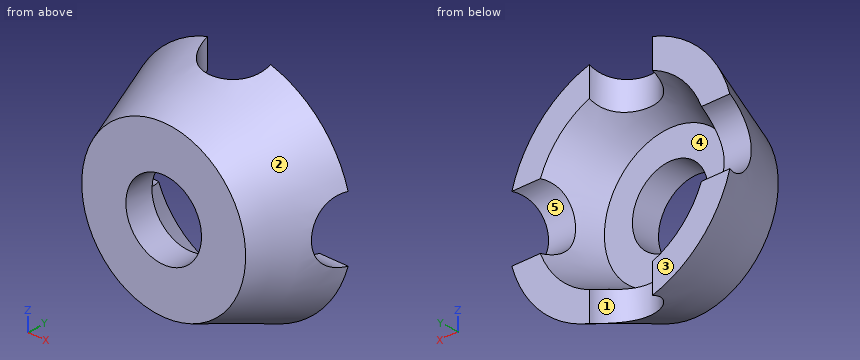
```python
from build123d import *

# Parameters (mm, degrees)
CUT_EXTRUDE1_DEPTH      = 58.166423712
CUT_EXTRUDE1_DEPTH_BACK = 58.166423712
SKETCH11_R              = 10
CUT_EXTRUDE2_DEPTH      = 57.284989289
CUT_EXTRUDE2_DEPTH_BACK = 57.284989289
SKETCH12_R              = 10
SKETCH13_R              = 12
CUT_EXTRUDE3_DEPTH      = 26


with BuildPart() as part:
    # Sketch9 → Revolve2 (revolve)
    with BuildSketch(Plane.XY, mode=Mode.PRIVATE) as revolve2_sk:
        Polygon((0, 9), (0, 0), (26, 0), (36, 26), (27.428684137, 26), (20.890222599, 9), align=None)
    revolve(revolve2_sk.sketch.rotate(Axis((0, 0, 0), (0, 1, 0)), 90), axis=Axis((0, 0, 0), (0, 1, 0)))

    # Sketch11 → Cut-Extrude1 (cut, two sides: drawn at the far end of the back side and taken through both)
    with BuildSketch(Plane.XY.offset(-CUT_EXTRUDE1_DEPTH_BACK)):
        with Locations((0, 26)):
            Circle(SKETCH11_R)
    extrude(amount=CUT_EXTRUDE1_DEPTH + CUT_EXTRUDE1_DEPTH_BACK, mode=Mode.SUBTRACT)

    # Sketch12 → Cut-Extrude2 (cut, two sides: drawn at the far end of the back side and taken through both)
    with BuildSketch(Plane(origin=(0, 0, 0), x_dir=(0, 0, -1), z_dir=(1, 0, 0)).offset(-CUT_EXTRUDE2_DEPTH_BACK)):
        with Locations((0, 26)):
            Circle(SKETCH12_R)
    extrude(amount=CUT_EXTRUDE2_DEPTH + CUT_EXTRUDE2_DEPTH_BACK, mode=Mode.SUBTRACT)

    # Sketch13 → Cut-Extrude3 (cut)
    with BuildSketch(Plane(origin=(0, 9, 0), x_dir=(1, 0, 0), z_dir=(0, 1, 0))):
        with Locations(Location((0, 0, 0), (0, 0, 270))):
            Circle(SKETCH13_R)
    extrude(amount=-CUT_EXTRUDE3_DEPTH, mode=Mode.SUBTRACT)


solid = part.part
```
Can you work these out from the model? Positions are in its coordinate system, mm. Face numbers are marked on the shaded views. A direction names the side the tool comes from. Round coordinates to 2 decimals unless told otherwise and drop trailing zeros. Order: outer loops, then holes, each group sorted by start corner. A loop starts at its lowest first (then second) coordinate and runs counter-clockwise, first axis right, second up.
(1) I'm going to push flat-ended pins straight in: pin 1 (5 mm diameter, centred on y = 16.5, z = 26.5, fed in from -X); pin 2 (19 mm diameter, centred on x = 0, z = 0, fed in from -Y); pin 3 (10 mm diameter, centred on y = 6, z = -9.5, fed in from -X); pin 4 (21 mm diameter, centred on x = -7.5, z = -2, fed in from +Y). Where does each tip first touch, or does it pass through?
Results are:
pin 1: stops at x = -22.04
pin 2: passes through
pin 3: stops at x = -29.14
pin 4: stops at y = 9
(2) If we section it at B-B (z = 0): Please give me the cut outline in (x, y).
Results are:
outline: (-32.15, 16) - (-26, 0) - (-12, 0) - (-12, 9) - (-20.89, 9) - (-23.58, 16) - close; (12, 0) - (26, 0) - (32.15, 16) - (23.58, 16) - (20.89, 9) - (12, 9) - close
(3) If we section it at C-C (y = 3.25): Please give me the cut outline in (x, z).
Results are:
outline: circle Ø54.5 at (0, 0); hole circle Ø24 at (0, 0)
(4) We'd pull the mould along X, two halves only. Please class the marked faces 1, 2 and 3: +X half, -X half, draft (parallel to the pull), parting line (faces both ways), or undercut.
Results are:
face 1: undercut
face 2: parting line
face 3: draft
(5) On a 3-axis mill with a long thin cutter (end or side, diameter ignored), from which of +Z, -Z, +X, -X, +Y, -Y can I reach the whole of each face in a straight line? I mean the marked faces 4 and 5. Say none if no direction works.
Results are:
face 4: +Y
face 5: +X, -X, +Y
(6) If we section it at A-A (x = 0): Please give me the cut outline in (y, z).
Results are:
outline: (0, -26) - (16, -32.15) - (16, -23.58) - (9, -20.89) - (9, -12) - (0, -12) - close; (0, 12) - (9, 12) - (9, 20.89) - (16, 23.58) - (16, 32.15) - (0, 26) - close
(7) If I drill on L1, parallel to Y at x = -13, z = 1.5; L2, parallel to X at y = 14.5, z = -14.5; L3, parallel to Z at x = -2.5, y = 1.75, over which ranges is the centre line in solid material (lowest first)?
Results are:
L1: y = 0 to 9
L2: x = -28.05 to -17.86, 17.86 to 28.05
L3: z = -26.56 to -11.74, 11.74 to 26.56
